```python
from build123d import *

# Parameters (mm, degrees)
F0_W      = 36
F0_H      = 6
F0_W_2    = 12
F0_H_2    = 3
F0_W_3    = 34
F0_W_4    = 2.5
F0_H_3    = 40
F1_DEPTH  = 2
F2_W      = 5
F2_H      = 1.5
F2_W_2    = 1.5
F2_H_2    = 6
F3_DEPTH  = 11
F4_W      = 5
F4_H      = 1.5
F5_DEPTH  = 4
F6_W      = 6
F6_H      = 1.5
F7_DEPTH  = 9
F8_W      = 6
F8_H      = 1.5
F9_DEPTH  = 9
F10_W     = 12
F10_H     = 12
F11_DEPTH = 8
F12_R     = 5
F13_DEPTH = 6
F15_DEPTH = 10
F16_R     = 2.99999
F17_R     = 2


# Not quite as in the source:
# - a fillet or chamfer is up to 0.001 mm smaller than in the source, because OpenCascade refuses the exact size


with BuildPart() as f1:
    # F0 (on Top) → F1 (new body)
    with BuildSketch(Plane.XY):
        with Locations((64, 0)):
            Rectangle(F0_W, F0_H)
        Polygon((46, -3), (46, 3), (34, 3), (34, 0), (34, -3), align=None)
        with Locations((40, 4.5)):
            Rectangle(F0_W_2, F0_H_2)
        Polygon((34, 0), (34, 3), (-34, 3), (-34, 0), (0, 0), align=None)
        Polygon((46, -6), (46, -3), (34, -3), (34, -6), (37.5, -6), (40, -6), (42.5, -6), align=None)
        Polygon((-34, 0), (-34, 3), (-46, 3), (-46, -3), (-34, -3), align=None)
        with Locations((-40, 4.5)):
            Rectangle(F0_W_2, F0_H_2)
        with Locations((17, -1.5)):
            Rectangle(F0_W_3, F0_H_2)
        with Locations((-64, 0)):
            Rectangle(F0_W, F0_H)
        with Locations((-17, -1.5)):
            Rectangle(F0_W_3, F0_H_2)
        with Locations((41.25, -26)):
            Rectangle(F0_W_4, F0_H_3)
        Polygon((-34, -3), (-46, -3), (-46, -6), (-42.5, -6), (-40, -6), (-37.5, -6), (-34, -6), align=None)
        with Locations((38.75, -26)):
            Rectangle(F0_W_4, F0_H_3)
        with Locations((-41.25, -26)):
            Rectangle(F0_W_4, F0_H_3)
        with Locations((-38.75, -26)):
            Rectangle(F0_W_4, F0_H_3)
    extrude(amount=F1_DEPTH)

    # F2 (on face) → F3 (join)
    with BuildSketch(Plane.XY.offset(2)):
        with Locations((-40, -45.25)):
            Rectangle(F2_W, F2_H)
        with Locations((40, -45.25)):
            Rectangle(F2_W, F2_H)
        with Locations((-81.25, 0)):
            Rectangle(F2_W_2, F2_H_2)
        with Locations((81.25, 0)):
            Rectangle(F2_W_2, F2_H_2)
    extrude(amount=F3_DEPTH)

    # F4 (on face) → F5 (join)
    with BuildSketch(Plane(origin=(0, -44.5, 0), x_dir=(-1, 0, 0), z_dir=(0, 1, 0))):
        with Locations((40, 12.25)):
            Rectangle(F4_W, F4_H)
        with Locations((-40, 12.25)):
            Rectangle(F4_W, F4_H)
    extrude(amount=F5_DEPTH)

    # F6 (on face) → F7 (join)
    with BuildSketch(Plane(origin=(80.5, 0, 0), x_dir=(0, -1, 0), z_dir=(-1, 0, 0))):
        with Locations((0, 12.25)):
            Rectangle(F6_W, F6_H)
    extrude(amount=F7_DEPTH)

    # F8 (on face) → F9 (join)
    with BuildSketch(Plane.YZ.offset(-80.5)):
        with Locations((0, 12.25)):
            Rectangle(F8_W, F8_H)
    extrude(amount=F9_DEPTH)

    # F10 (on face) → F11 (join)
    with BuildSketch(Plane(origin=(0, 0, 0), x_dir=(1, 0, 0), z_dir=(0, 0, -1))):
        with Locations((-40, 0)):
            Rectangle(F10_W, F10_H)
        with Locations((40, 0)):
            Rectangle(F10_W, F10_H)
    extrude(amount=F11_DEPTH)

    # F12 (on face) → F13 (cut)
    with BuildSketch(Plane.XY.offset(2)):
        with Locations((-40, 0)):
            Circle(F12_R)
        with Locations((40, 0)):
            Circle(F12_R)
    extrude(amount=-F13_DEPTH, mode=Mode.SUBTRACT)

    # F14 (on face) → F15 (cut)
    with BuildSketch(Plane(origin=(0, 0, -8), x_dir=(1, 0, 0), z_dir=(0, 0, -1))):
        with BuildLine():
            ThreePointArc((42.8284271247, -1), (42.956795679, -0.5073059362), (43, 0))
            ThreePointArc((43, 0), (42.956795679, 0.5073059362), (42.8284271247, 1))
            ThreePointArc((42.8284271247, 1), (42.1213203436, 2.1213203436), (41, 2.8284271247))
            ThreePointArc((41, 2.8284271247), (40, 3), (39, 2.8284271247))
            ThreePointArc((39, 2.8284271247), (37.8786796564, 2.1213203436), (37.1715728753, 1))
            ThreePointArc((37.1715728753, 1), (37, 0), (37.1715728753, -1))
            ThreePointArc((37.1715728753, -1), (37.8786796564, -2.1213203436), (39, -2.8284271247))
            ThreePointArc((39, -2.8284271247), (40, -3), (41, -2.8284271247))
            ThreePointArc((41, -2.8284271247), (42.1213203436, -2.1213203436), (42.8284271247, -1))
        make_face()
        with BuildLine():
            ThreePointArc((42.8284271247, 1), (42.956795679, 0.5073059362), (43, 0))
            ThreePointArc((43, 0), (42.956795679, -0.5073059362), (42.8284271247, -1))
            Line((42.8284271247, -1), (45, -1))
            Line((45, -1), (45, 0))
            Line((45, 0), (45, 1))
            Line((45, 1), (42.8284271247, 1))
        make_face()
        with BuildLine():
            ThreePointArc((39, 2.8284271247), (40, 3), (41, 2.8284271247))
            Line((41, 2.8284271247), (41, 5))
            Line((41, 5), (40, 5))
            Line((40, 5), (39, 5))
            Line((39, 5), (39, 2.8284271247))
        make_face()
        with BuildLine():
            Line((41, -5), (41, -2.8284271247))
            ThreePointArc((41, -2.8284271247), (40, -3), (39, -2.8284271247))
            Line((39, -2.8284271247), (39, -5))
            Line((39, -5), (40, -5))
            Line((40, -5), (41, -5))
        make_face()
        with BuildLine():
            ThreePointArc((37.1715728753, -1), (37, 0), (37.1715728753, 1))
            Line((37.1715728753, 1), (35, 1))
            Line((35, 1), (35, 0))
            Line((35, 0), (35, -1))
            Line((35, -1), (37.1715728753, -1))
        make_face()
        with BuildLine():
            ThreePointArc((-37.1715728753, -1), (-37.043204321, -0.5073059362), (-37, 0))
            ThreePointArc((-37, 0), (-37.043204321, 0.5073059362), (-37.1715728753, 1))
            ThreePointArc((-37.1715728753, 1), (-37.8786796564, 2.1213203436), (-39, 2.8284271247))
            ThreePointArc((-39, 2.8284271247), (-40, 3), (-41, 2.8284271247))
            ThreePointArc((-41, 2.8284271247), (-42.1213203436, 2.1213203436), (-42.8284271247, 1))
            ThreePointArc((-42.8284271247, 1), (-43, 0), (-42.8284271247, -1))
            ThreePointArc((-42.8284271247, -1), (-42.1213203436, -2.1213203436), (-41, -2.8284271247))
            ThreePointArc((-41, -2.8284271247), (-40, -3), (-39, -2.8284271247))
            ThreePointArc((-39, -2.8284271247), (-37.8786796564, -2.1213203436), (-37.1715728753, -1))
        make_face()
        with BuildLine():
            ThreePointArc((-37.1715728753, 1), (-37.043204321, 0.5073059362), (-37, 0))
            ThreePointArc((-37, 0), (-37.043204321, -0.5073059362), (-37.1715728753, -1))
            Line((-37.1715728753, -1), (-35, -1))
            Line((-35, -1), (-35, 0))
            Line((-35, 0), (-35, 1))
            Line((-35, 1), (-37.1715728753, 1))
        make_face()
        with BuildLine():
            ThreePointArc((-41, 2.8284271247), (-40, 3), (-39, 2.8284271247))
            Line((-39, 2.8284271247), (-39, 5))
            Line((-39, 5), (-40, 5))
            Line((-40, 5), (-41, 5))
            Line((-41, 5), (-41, 2.8284271247))
        make_face()
        with BuildLine():
            Line((-39, -5), (-39, -2.8284271247))
            ThreePointArc((-39, -2.8284271247), (-40, -3), (-41, -2.8284271247))
            Line((-41, -2.8284271247), (-41, -5))
            Line((-41, -5), (-40, -5))
            Line((-40, -5), (-39, -5))
        make_face()
        with BuildLine():
            ThreePointArc((-42.8284271247, -1), (-43, 0), (-42.8284271247, 1))
            Line((-42.8284271247, 1), (-45, 1))
            Line((-45, 1), (-45, 0))
            Line((-45, 0), (-45, -1))
            Line((-45, -1), (-42.8284271247, -1))
        make_face()
    extrude(amount=-F15_DEPTH, mode=Mode.SUBTRACT)

    # F16 (radius 3 in the source; OpenCascade refuses exactly that, so slightly less here)
    f16_edges = [f1.edges().sort_by_distance(p)[0] for p in [
        (-46, 6, -3),
        (-34, 6, -3),
        (-34, -6, -3),
        (-46, -6, -3),
        (46, 6, -3),
        (34, 6, -3),
        (46, -6, -3),
        (34, -6, -3),
        (40, -46, 0),
        (-40, -46, 0),
        (-82, 0, 0),
        (82, 0, 0),
    ]]
    fillet(f16_edges, radius=F16_R)

    # F17
    f17_edges = [f1.edges().sort_by_distance(p)[0] for p in [
        (-82, 0, 13),
        (-40, -46, 13),
        (40, -46, 13),
        (82, 0, 13),
    ]]
    fillet(f17_edges, radius=F17_R)


solid = f1.part
```
Here's how the part is built. I have some questions about the finished solid (model axes, mm). A direction names the side the tool comes from. Coordinates: 2 decimals unless noted, no trailing zeros. Order: outer loops, then holes, each group sorted by start corner. A loop starts at its lowest first (then second) coordinate and runs counter-clockwise, first axis right, second up.
1) Imagine slicing it at D-D on x = 49. List the corners of the cut face in (y, z) for me.
2) Imagine slicing it at B-B on z = 5.5. List the corners of the cut face in (x, y) for me, and give its area (3 significant figures).
3) I need wall thicknesses on line 1 (X direction, y = 0.5, z = -0.5); line 2 (X direction, y = -29, z = 0.25); line 3 (X direction, y = 0.5, z = 9.5). Which ranges of each line are inside material? Lowest first, please.
4) Imagine slicing it at C-C on z = -5.5. State how many separate pieces and enclosed holes the cut face has, and give its area (3 significant figures).
5) Will these pins go through, and if not, where does the flat tip stop? pin 1 (3 mm diameter, centred on x = 42.5, y = 2.5, fed in from +Z); pin 2 (6 mm diameter, centred on x = -23, z = 5.5, fed in from +Y); pin 3 (1.2 mm diameter, centred on x = 40, z = 12, fed in from +Y); pin 4 (3 mm diameter, centred on x = -39, z = -4, fed in from -Y).
6) Imagine slicing it at A-A on y = -12.5. List the corners of the cut face in (x, z) for me.
7) Which directions (+Z, -Z, +X, -X, +Y, -Y) give clear straight access to the entire face, cutting with the end or side of a thin tool? Please do faces 4 (the face through (-46, 0, -4)), 5 (the face through (68.1, 3, 1.7)), 6 (the face through (43, 3, -4)).
8) We'd pull the mould along X, two halves only. Please class faces 1 (the face through (-42.5, -29.1, 1.7)), 2 (the face through (34.9, 5.14, -3.07)), 3 (the face through (45.14, -5.1, -3.07)): +X half, -X half, draft (parallel to the pull), parting line (faces both ways), or undercut.
Response values:
1. outline: (-3, 0) - (3, 0) - (3, 2) - (-3, 2) - close
2. outline: (-82, -3) - (-80.5, -3) - (-80.5, 3) - (-82, 3) - close; (-42.5, -46) - (-37.5, -46) - (-37.5, -44.5) - (-42.5, -44.5) - close; (37.5, -46) - (42.5, -46) - (42.5, -44.5) - (37.5, -44.5) - close; (80.5, -3) - (82, -3) - (82, 3) - (80.5, 3) - close
2. area: 33.0 mm2
3. line 1: x = -46 to -45, -35 to -34, 34 to 35, 45 to 46
3. line 2: x = -42.5 to -37.5, 37.5 to 42.5
3. line 3: x = -82 to -80.5, 80.5 to 82
4. separate pieces: 2
4. enclosed holes: 2
4. area: 183 mm2
5. pin 1: stops at z = 2
5. pin 2: passes through
5. pin 3: stops at y = -40.5
5. pin 4: stops at y = -6
6. outline: (-42.5, 0) - (-37.5, 0) - (-37.5, 2) - (-42.5, 2) - close; (37.5, 0) - (42.5, 0) - (42.5, 2) - (37.5, 2) - close
7. face 4: -Z, -X, +Y, -Y
7. face 5: +Z, -Z, +X, +Y
7. face 6: +Z
8. face 1: -X half
8. face 2: undercut
8. face 3: +X half
